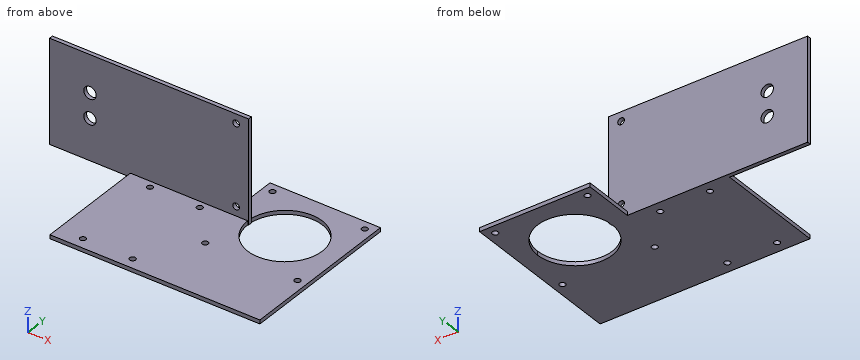
from build123d import *

# Parameters (mm, degrees)
SKETCH1_R           = 1.5
SKETCH1_R_2         = 19.05
BOSS_EXTRUDE1_DEPTH = 2
BOSS_EXTRUDE2_DEPTH = 52.8
SKETCH3_R           = 1.7
CUT_EXTRUDE1_DEPTH  = 133.22344724
SKETCH4_R           = 3.175
CUT_EXTRUDE2_DEPTH  = 10


with BuildPart() as part:
    # Sketch1 → Boss-Extrude1 (new body)
    with BuildSketch(Plane.XY):
        Polygon((0, 58.4), (0, 0), (107.2, 0), (107.2, 84.53204182), (50.8, 84.53204182), (50.8, 58.4), align=None)
        with Locations((102.55, 79.88204182)):
            Circle(SKETCH1_R, mode=Mode.SUBTRACT)
        with Locations((102.55, 32.78204182)):
            Circle(SKETCH1_R, mode=Mode.SUBTRACT)
        with Locations((55.45, 32.78204182)):
            Circle(SKETCH1_R, mode=Mode.SUBTRACT)
        with Locations((55.45, 79.88204182)):
            Circle(SKETCH1_R, mode=Mode.SUBTRACT)
        with Locations((12.7, 52.75)):
            Circle(SKETCH1_R, mode=Mode.SUBTRACT)
        with Locations((38.1, 52.75)):
            Circle(SKETCH1_R, mode=Mode.SUBTRACT)
        with Locations((12.7, 5.65)):
            Circle(SKETCH1_R, mode=Mode.SUBTRACT)
        with Locations((38.1, 5.65)):
            Circle(SKETCH1_R, mode=Mode.SUBTRACT)
        with Locations((79, 56.33204182)):
            Circle(SKETCH1_R_2, mode=Mode.SUBTRACT)
    extrude(amount=-BOSS_EXTRUDE1_DEPTH)

    # Sketch2 → Boss-Extrude2 (add)
    with BuildSketch(Plane(origin=(0, 0, -2), x_dir=(-1, 0, 0), z_dir=(0, 0, -1))):
        Polygon((0, 58.4), (41.275, 58.4), (41.275, 56.4), (0, 56.4), (-60.325, 56.4), (-60.325, 58.4), align=None)
    extrude(amount=-BOSS_EXTRUDE2_DEPTH)

    # Sketch3 → Cut-Extrude1 (cut, through all)
    with BuildSketch(Plane(origin=(0, 58.4, 0), x_dir=(1, 0, 0), z_dir=(0, 1, 0))):
        with Locations(Location((53.975, -4.7625, 0), (0, 0, 180))):
            Circle(SKETCH3_R)
        with Locations(Location((53.975, -46.0375, 0), (0, 0, 180))):
            Circle(SKETCH3_R)
    extrude(amount=-CUT_EXTRUDE1_DEPTH, mode=Mode.SUBTRACT)

    # Sketch4 → Cut-Extrude2 (cut)
    with BuildSketch(Plane(origin=(0, 58.4, 0), x_dir=(1, 0, 0), z_dir=(0, 1, 0))):
        with Locations(Location((-20.6375, -19.05, 0), (0, 0, 180))):
            Circle(SKETCH4_R)
        with Locations(Location((-20.6375, -31.75, 0), (0, 0, 180))):
            Circle(SKETCH4_R)
    extrude(amount=-CUT_EXTRUDE2_DEPTH, mode=Mode.SUBTRACT)


solid = part.part
Work out the finished part from the listing and answer in its coordinate system (mm). Round coordinates to 2 decimals unless told otherwise and drop trailing zeros. Write each loop counter-clockwise with the first axis right and the second up, starting at its lowest first coordinate (ties: lowest second). Pieces come first, ordered by that corner, then holes.
1) A cutting plane is placed at A-A (z = 19.05). Give the vertices of the cut face in (x, y) (1 decimal).
2) A cutting plane is placed at C-C (y = 52.75). Give the vertices of the cut face in (x, z), plus the area to 3 significant figures.
3) A cutting plane is placed at D-D (y = 68). Give the vertices of the cut face in (x, z), plus the area to 3 significant figures.
4) Given pin 1 Ø2.5 at (x, y) = (38.1, 52.75) entering from +Z; pin 2 Ø5 at (x, y) = (12.7, 5.65) entering from +Z; pin 3 Ø3 at (x, z) = (9, 32.5) entering from -Y; pin 4 Ø2 at (y, z) = (21, -0.5) entering from -X, each flat-ended and moving along its own axis, determine where each tip first touches the part or whether it passes through.
5) A cutting plane is placed at B-B (x = 12.7). Give the vertices of the cut face in (y, z).
6) Straight lines are drawn through the part: line 1 (Y direction, x = 55.45, z = -0.45); line 2 (Y direction, x = 38, z = -1); line 3 (Z direction, x = 53.5, y = 57.5). For each, find the intervals that lie inside material, in ascending order.
Completed:
1. outline: (-41.3, 56.4) - (-23.8, 56.4) - (-23.8, 58.4) - (-41.3, 58.4) - close; (-17.5, 56.4) - (60.3, 56.4) - (60.3, 58.4) - (-17.5, 58.4) - close
2. outline: (0, -2) - (11.2, -2) - (11.2, 0) - (0, 0) - close; (14.2, -2) - (36.6, -2) - (36.6, 0) - (14.2, 0) - close; (39.6, -2) - (60.29, -2) - (60.29, 0) - (39.6, 0) - close; (97.71, -2) - (107.2, -2) - (107.2, 0) - (97.71, 0) - close
2. area: 128 mm2
3. outline: (50.8, -2) - (63.94, -2) - (63.94, 0) - (50.8, 0) - close; (94.06, -2) - (107.2, -2) - (107.2, 0) - (94.06, 0) - close
3. area: 52.6 mm2
4. pin 1: passes through
4. pin 2: stops at z = 0
4. pin 3: stops at y = 56.4
4. pin 4: stops at x = 0
5. outline: (0, -2) - (4.15, -2) - (4.15, 0) - (0, 0) - close; (7.15, -2) - (51.25, -2) - (51.25, 0) - (7.15, 0) - close; (54.25, -2) - (58.4, -2) - (58.4, 50.8) - (56.4, 50.8) - (56.4, 0) - (54.25, 0) - close
6. line 1: y = 0 to 31.28, 34.28 to 78.38, 81.38 to 84.53
6. line 2: y = 0 to 4.15, 7.15 to 51.25, 54.25 to 58.4
6. line 3: z = -2 to 3.13, 6.39 to 44.41, 47.67 to 50.8
